Work out the finished part from the listing and answer in its coordinate system (mm). A direction names the side the tool comes from. Coordinates: 2 decimals unless noted, no trailing zeros. Order: outer loops, then holes, each group sorted by start corner. A loop starts at its lowest first (then second) coordinate and runs counter-clockwise, first axis right, second up. Notation, with made-up numbers: M 55.5,88.25 L 95.5,88.25 A36 ccw 95.5,127.25 Z; hole C 86,3 d2. An arc over 180 degrees is marked long. Use a Markdown table: item, result.
from build123d import *

# Parameters (mm, degrees)
SKETCH2_R                 = 145
SKETCH2_R_2               = 105
BOSS_EXTRUDE1_START       = -50
SKETCH3_W                 = 360
SKETCH3_H                 = 360
SKETCH3_R                 = 145
BOSS_EXTRUDE1_DEPTH       = 50
FILLET1_R                 = 20
SKETCH4_R                 = 145
BOSS_EXTRUDE2_DEPTH       = 50
SKETCH5_R                 = 30
CUT_EXTRUDE2_DEPTH        = 10
CUT_EXTRUDE3_REACH        = 719.763
SKETCH6_R                 = 15
CIRPATTERN1_COUNT         = 4
SKETCH7_R                 = 30
CUT_EXTRUDE4_DEPTH        = 10
SKETCH8_R                 = 15
CUT_EXTRUDE5_DEPTH        = 829.171628686
CIRPATTERN4_START         = 332.601345058
CIRPATTERN4_OUTLINE_R     = 15
CIRPATTERN4_DEPTH         = 50
CIRPATTERN4_START_2       = 372.601345058
CIRPATTERN4_2_OUTLINE_R   = 30
CIRPATTERN4_2_OUTLINE_R_2 = 15
CIRPATTERN4_2_DEPTH       = 10
CHAMFER1_SIZE             = 10


# Read off the part's stored shape, not the designer's step: CirPattern4
with BuildPart() as part:
    # Sweep-Thin1: sweep along a path in Sketch1
    with BuildLine(Plane.XY) as sweep_thin1_path:
        Line((0, 0), (-150, 0))
        ThreePointArc((-150, 0), (-333.847763109, 76.152236891), (-410, 260))
        Line((-410, 260), (-410, 382.601345058))
    # Sketch2 → Sweep-Thin1 (sweep)
    with BuildSketch(Plane(origin=(0, 0, 0), x_dir=(0, 0, -1), z_dir=(1, 0, 0))):
        Circle(SKETCH2_R)
        Circle(SKETCH2_R_2, mode=Mode.SUBTRACT)
    sweep(path=sweep_thin1_path.line)

    # Sketch3 → Boss-Extrude1 (add)
    with BuildSketch(Plane(origin=(0, 0, 0), x_dir=(0, 0, -1), z_dir=(1, 0, 0)).offset(BOSS_EXTRUDE1_START)):
        Rectangle(SKETCH3_W, SKETCH3_H)
        with Locations(Location((0, 0, 0), (0, 0, 270))):
            Circle(SKETCH3_R, mode=Mode.SUBTRACT)
    extrude(amount=BOSS_EXTRUDE1_DEPTH)

    # Fillet1
    fillet1_edges = [part.edges().sort_by_distance(p)[0] for p in [
        (-25, -180, -180),
        (-25, -180, 180),
        (-25, 180, 180),
        (-25, 180, -180),
    ]]
    fillet(fillet1_edges, radius=FILLET1_R)

    # Sketch4 → Boss-Extrude2 (add)
    with BuildSketch(Plane(origin=(0, 382.601345058, 0), x_dir=(1, 0, 0), z_dir=(0, 1, 0))):
        with BuildLine():
            Line((-570, -180), (-250, -180))
            ThreePointArc((-250, -180), (-235.857864376, -174.142135624), (-230, -160))
            Line((-230, -160), (-230, 160))
            ThreePointArc((-230, 160), (-235.857864376, 174.142135624), (-250, 180))
            Line((-250, 180), (-570, 180))
            ThreePointArc((-570, 180), (-584.142135624, 174.142135624), (-590, 160))
            Line((-590, 160), (-590, -160))
            ThreePointArc((-590, -160), (-584.142135624, -174.142135624), (-570, -180))
        make_face()
        with Locations(Location((-410, 0, 0), (0, 0, 180))):
            Circle(SKETCH4_R, mode=Mode.SUBTRACT)
    extrude(amount=-BOSS_EXTRUDE2_DEPTH)

    # Sketch5 → Cut-Extrude2 (cut)
    with BuildSketch(Plane(origin=(0, 0, 0), x_dir=(0, 0, -1), z_dir=(1, 0, 0))):
        with Locations((-130, 130)):
            Circle(SKETCH5_R)
    cut_extrude2 = extrude(amount=-CUT_EXTRUDE2_DEPTH, mode=Mode.SUBTRACT)

    # Sketch6 → Cut-Extrude3 (cut, up to next)
    with BuildSketch(Plane(origin=(-10, 0, 0), x_dir=(0, 0, -1), z_dir=(1, 0, 0)), mode=Mode.PRIVATE) as cut_extrude3_sk1:
        with Locations((-130, 130)):
            Circle(SKETCH6_R)
    cut_extrude3_tool1 = extrude(cut_extrude3_sk1.sketch, amount=-CUT_EXTRUDE3_REACH, mode=Mode.PRIVATE) & part.part
    cut_extrude3 = cut_extrude3_tool1.solids().sort_by_distance((-10, 130, 130))[0]
    add(cut_extrude3, mode=Mode.SUBTRACT)

    # CirPattern1: Cut-Extrude2, Cut-Extrude3 ×4 about axis
    cirpattern1_axis = Axis((0, 0, 0), (1, 0, 0))
    add([cut_extrude2.rotate(cirpattern1_axis, i * 360 / CIRPATTERN1_COUNT) for i in range(1, CIRPATTERN1_COUNT)], mode=Mode.SUBTRACT)
    add([cut_extrude3.rotate(cirpattern1_axis, i * 360 / CIRPATTERN1_COUNT) for i in range(1, CIRPATTERN1_COUNT)], mode=Mode.SUBTRACT)

    # Sketch7 → Cut-Extrude4 (cut)
    with BuildSketch(Plane(origin=(0, 382.601345058, 0), x_dir=(1, 0, 0), z_dir=(0, 1, 0))):
        with Locations(Location((-540, -130, 0), (0, 0, 180))):
            Circle(SKETCH7_R)
    extrude(amount=-CUT_EXTRUDE4_DEPTH, mode=Mode.SUBTRACT)

    # Sketch8 → Cut-Extrude5 (cut, through all)
    with BuildSketch(Plane(origin=(0, 372.601345058, 0), x_dir=(1, 0, 0), z_dir=(0, 1, 0))):
        with Locations(Location((-540, -130, 0), (0, 0, 180))):
            Circle(SKETCH8_R)
    extrude(amount=-CUT_EXTRUDE5_DEPTH, mode=Mode.SUBTRACT)

    # CirPattern4 outline → CirPattern4 (cut)
    with BuildSketch(Plane(origin=(0, 0, 0), x_dir=(1, 0, 0), z_dir=(0, 1, 0)).offset(CIRPATTERN4_START)):
        with Locations((-280, -130)):
            Circle(CIRPATTERN4_OUTLINE_R)
        with Locations((-280, 130)):
            Circle(CIRPATTERN4_OUTLINE_R)
        with Locations((-540, 130)):
            Circle(CIRPATTERN4_OUTLINE_R)
    extrude(amount=CIRPATTERN4_DEPTH, mode=Mode.SUBTRACT)

    # CirPattern4 2 outline → CirPattern4 2 (cut)
    # profile 1 of 3: a face of its own
    with BuildSketch(Plane(origin=(0, 0, 0), x_dir=(1, 0, 0), z_dir=(0, 1, 0)).offset(CIRPATTERN4_START_2)):
        with Locations((-280, -130)):
            Circle(CIRPATTERN4_2_OUTLINE_R)
        with Locations((-280, -130)):
            Circle(CIRPATTERN4_2_OUTLINE_R_2, mode=Mode.SUBTRACT)
    # profile 2 of 3: a face of its own
    with BuildSketch(Plane(origin=(0, 0, 0), x_dir=(1, 0, 0), z_dir=(0, 1, 0)).offset(CIRPATTERN4_START_2)):
        with Locations((-280, 130)):
            Circle(CIRPATTERN4_2_OUTLINE_R)
        with Locations((-280, 130)):
            Circle(CIRPATTERN4_2_OUTLINE_R_2, mode=Mode.SUBTRACT)
    # profile 3 of 3: a face of its own
    with BuildSketch(Plane(origin=(0, 0, 0), x_dir=(1, 0, 0), z_dir=(0, 1, 0)).offset(CIRPATTERN4_START_2)):
        with Locations((-540, 130)):
            Circle(CIRPATTERN4_2_OUTLINE_R)
        with Locations((-540, 130)):
            Circle(CIRPATTERN4_2_OUTLINE_R_2, mode=Mode.SUBTRACT)
    extrude(amount=CIRPATTERN4_2_DEPTH, mode=Mode.SUBTRACT)

    # Chamfer1
    chamfer1_edges = [part.edges().sort_by_distance(p)[0] for p in [
        (0, 0, 105),
        (-410, 382.601345058, 105),
    ]]
    chamfer(chamfer1_edges, length=CHAMFER1_SIZE)


solid = part.part
(1) Straight lines are drawn through the part: L1, parallel to Y at x = -20.5, z = -130; L2, parallel to Z at x = -280, y = 375. For each, find the intervals that lie inside material, in ascending order.
Conclusion:
| item | result |
|---|---|
| L1 | -180 to -145, -115 to 115, 145 to 180 |
| L2 | -180 to -160, -100 to 100, 160 to 180 |
(2) A cutting plane is placed at C-C (y = 130). Give the number of separate pieces and of enclosed holes in the cut face, then the cut area to 3 significant figures.
Conclusion:
| item | result |
|---|---|
| separate pieces | 3 |
| enclosed holes | 1 |
| area | 71,600 mm2 |
(3) Given P1, Ø1, axis at x = -162.5, y = -21.5, coming from the +Z side; P2, Ø10, axis at y = 247.5, z = 67.5, coming from the -X side; P3, Ø18, axis at x = -271.5, z = -127, coming from the +Y side, each flat-ended and moving along its own axis, determine where each tip first touches the part or whether it passes through.
Conclusion:
| item | result |
|---|---|
| P1 | z = 143.43 |
| P2 | x = -540.64 |
| P3 | y = 372.6 |
(4) A cutting plane is placed at A-A (z = 0). Determine the outline of the cut face in (x, y).
Conclusion:
| item | result |
|---|---|
| outline | M -590,332.6 L -555,332.6 L -555,260 A405 ccw -150,-145 L -50,-145 L -50,-180 L 0,-180 L 0,-115 L -10,-105 L -150,-105 A365 cw -515,260 L -515,372.6 L -525,382.6 L -590,382.6 Z; M -305,260 A155 ccw -150,105 L -10,105 L 0,115 L 0,180 L -50,180 L -50,145 L -150,145 A115 cw -265,260 L -265,332.6 L -230,332.6 L -230,382.6 L -295,382.6 L -305,372.6 Z |
(5) Determine the mould class of faces 1 (the cylindrical face through (-265.693, 352.321, 125.494)), 2 (the flat face through (0, 83, 83)), 3 (the cylindrical face through (-100.7, -43.554, -138.304)) for opening direction Z: pulls with the +Z half, pulls with the -Z half, needs draft (parallel to the pull), parting line crosses it, or undercut.
Conclusion:
| item | result |
|---|---|
| face 1 | undercut |
| face 2 | needs draft |
| face 3 | parting line crosses it |
(6) A cutting plane is placed at B-B (x = -117.5). Determine the outline of the cut face in (y, z), then the cut area to 3 significant figures.
Conclusion:
| item | result |
|---|---|
| outline | C 0,0 d290; hole C 0,0 d210 |
| area | 31,400 mm2 |
(7) Which of the six approach directions +Z, -Z, +X, -X, +Y, -Y give full straight-line access (tool end or side, diameter ignored) to faces 4 (the cylindrical face through (-4.93, 100.713, 136.503)), 5 (the cylindrical face through (-265.693, 352.321, -134.506)), 6 (the cylindrical face through (-453.554, 296.809, -138.304))?
Conclusion:
| item | result |
|---|---|
| face 4 | +X |
| face 5 | +Y |
| face 6 | none |
